Geometry check sheet. Reference: the model listing, model coordinates, mm. A direction names the side the tool comes from. Give positions to 0.01 mm unless a question says otherwise; leave off trailing zeros. Loops run counter-clockwise (first coordinate to the right, second up) from the corner with the lowest first, then second, coordinate; pieces in that order, holes last.
1. Cross-section at A-A, the plane y = -96. Record the cut outline in (x, z).
2. Tool access check on faces 1 (the flat face through (-17, -152.4, -271)), 2 (the cylindrical face through (-5.506, 79.261, -278.796)). Record the directions out of +Z, -Z, +X, -X, +Y, -Y that give a thin tool (end or side, any length) a straight path to the whole face; none if there is none.
3. Cross-section at B-B, the plane x = -16.5. Record the cut outline in (y, z), plus the area to 3 significant figures.
4. Cross-section at C-C, the plane x = 8.5. Record the cut outline in (y, z).
5. Go/stop test with flat-tipped pins: pin 1 Ø5 at (x, z) = (5, -61) entering from +Y; pin 2 Ø1 at (x, z) = (-15, -61.5) entering from -Y; pin 3 Ø10 at (x, y) = (-14.5, 45) entering from -Z. Record where each tip stops, or that it passes through.
6. Release check for a two-part mould opening along Z. For faces 3 (the flat face through (-17, -152.4, 17)), 4 (the cylindrical face through (-18.846, 79.261, -268.451)), 5 (the cylindrical face through (22.652, 85.839, -7.134)) record: +Z half, -Z half, draft (parallel to the pull), parting line (faces both ways), or undercut.
7. Material ranges on L1, parallel to Z at x = 0, y = 203.5; L2, parallel to X at y = 205.5, z = 1.5; L3, parallel to Z at x = -12, y = 0, recorded low to high.
8. Cross-section at D-D, the plane y = 369. State how many separate pieces and enclosed holes the cut face has, plus the area to 3 significant figures.
from build123d import *

# Parameters (mm, degrees)
SKETCH2_R   = 25.4
SKETCH2_R_2 = 23.749


with BuildPart() as part:
    # Sweep1: sweep along a path in Sketch1
    with BuildLine(Plane(origin=(0, 0, 0), x_dir=(0, 0, -1), z_dir=(1, 0, 0))) as sweep1_path:
        Line((0, -152.4), (0, 0))
        Line((0, 0), (0, 317.5))
        ThreePointArc((0, 317.5), (127, 444.5), (254, 317.5))
        Line((254, 317.5), (254, 0))
        Line((254, 0), (254, -152.4))
    # Sketch2 → Sweep1 (sweep)
    with BuildSketch(Plane(origin=(0, -152.4, 0), x_dir=(1, 0, 0), z_dir=(0, 1, 0))):
        Circle(SKETCH2_R)
        Circle(SKETCH2_R_2, mode=Mode.SUBTRACT)
    sweep(path=sweep1_path.line)


solid = part.part
Result:
1. outline: circle Ø50.8 at (0, -254); circle Ø50.8 at (0, 0); hole circle Ø47.5 at (0, -254); hole circle Ø47.5 at (0, 0)
2. face 1: +Z, -Z, +X, -X, -Y
2. face 2: -Y
3. outline: (-152.4, -273.31) - (317.5, -273.31) arc R146.31 ccw to (317.5, 19.31) - (-152.4, 19.31) - (-152.4, 17.08) - (317.5, 17.08) arc R144.08 cw to (317.5, -271.08) - (-152.4, -271.08) - close; (-152.4, -236.92) - (317.5, -236.92) arc R109.92 ccw to (317.5, -17.08) - (-152.4, -17.08) - (-152.4, -19.31) - (317.5, -19.31) arc R107.69 cw to (317.5, -234.69) - (-152.4, -234.69) - close
3. area: 5,970 mm2
4. outline: (-152.4, -277.94) - (317.5, -277.94) arc R150.94 ccw to (317.5, 23.94) - (-152.4, 23.94) - (-152.4, 22.18) - (317.5, 22.18) arc R149.18 cw to (317.5, -276.18) - (-152.4, -276.18) - close; (-152.4, -231.82) - (317.5, -231.82) arc R104.82 ccw to (317.5, -22.18) - (-152.4, -22.18) - (-152.4, -23.94) - (317.5, -23.94) arc R103.06 cw to (317.5, -230.06) - (-152.4, -230.06) - close
5. pin 1: stops at y = 455.6
5. pin 2: stops at y = 400.88
5. pin 3: stops at z = -277.56
6. face 3: draft
6. face 4: undercut
6. face 5: undercut
7. L1: z = -279.4 to -277.75, -230.25 to -228.6, -25.4 to -23.75, 23.75 to 25.4
7. L2: x = -25.36 to -23.7, 23.7 to 25.36
7. L3: z = -276.39 to -274.49, -233.51 to -231.61, -22.39 to -20.49, 20.49 to 22.39
8. separate pieces: 2
8. enclosed holes: 2
8. area: 562 mm2
